Input: part model. Units: mm. Frame: model coordinates. A direction names the side the tool comes from. Coordinates: 2 decimals unless noted, no trailing zeros. Order: outer loops, then holes, each group sorted by start corner. A loop starts at its lowest first (then second) coordinate and runs counter-clockwise, first axis right, second up. Notation, with made-up numbers: (-13.5, -27) -> (21.5, -27) arc R13 ccw to (21.5, -21) -> close; hole circle Ø5 at (47, 39). An arc over 180 degrees is marked (long way). Use one line per item in the form item = value. Start each with the question number.
1) Ray query, line 1 along X through (y, z) = (54, 203); line 2 along Z through (x, y) = (-20, 92); line 3 along Y through (x, z) = (-42.5, -67). Return the intervals inside material, ascending.
2) Pin query (flat end, axial travel): pin 1 (15 mm diameter, centred on x = 118.06, z = -176.69, fed in from +Y); pin 2 (15 mm diameter, centred on x = -41.46, z = 208.42, fed in from -Y); pin 3 (1 mm diameter, centred on y = -22, z = -51, fed in from -X); pin 4 (10.5 mm diameter, centred on x = -41.46, z = -208.42, fed in from +Y). Return the tip coordinate at first contact, or that it passes through.
3) Access query for faces 4 (the flat face through (-188.79, 53.307, -105.435)), 5 (the conical face through (-81.465, 47.154, -197.721)), 6 (the cylindrical face through (-143.719, 61.042, 143.366)), 7 (the flat face through (105.7, 53.31, 188.99)). Directions: +Z, -Z, +X, -X, +Y, -Y. A direction counts if a zero-diameter tool reaches every point of the face in a straight line with its end or side. Return the directions, or none.
4) Section query C-C on y = 101. Output: boundary loops of the cut face in (x, z), then the cut area to 3 significant figures.
5) Draft query along X for faces 1 (the cylindrical face through (-187.452, 61.042, -77.915)), 2 (the conical face through (197.721, 47.154, -81.465)), 3 (the conical face through (0, 47, 214)). Return one class per face: pulls with the +X half, pulls with the -X half, needs draft (parallel to the pull), parting line crosses it, or undercut.
from build123d import *

# Parameters (mm, degrees)
CUT_EXTRUDE1_DEPTH = 28
CIRPATTERN1_COUNT  = 16
SKETCH5_R          = 6.5
CUT_EXTRUDE2_DEPTH = 336.079515181
CHAMFER1_SIZE      = 2


with BuildPart() as part:
    # Sketch1 → Revolve1 (revolve)
    with BuildSketch(Plane.XY, mode=Mode.PRIVATE) as revolve1_sk:
        Polygon((225, 0), (225, 64), (202.5, 64), (200, 95.5), (180, 95.5), (180, 123.5), (143, 123.5), (143, 88.5), (85, 88.5), (85, 116.5), (66, 116.5), (66, -41.015625), (86.5078125, -41.015625), (86.5078125, 0), align=None)
    revolve(revolve1_sk.sketch.rotate(Axis((0, 0, 0), (0, 1, 0)), 90), axis=Axis((0, 0, 0), (0, 1, 0)))

    # Sketch3 → Cut-Extrude1 (cut)
    with BuildSketch(Plane(origin=(0, 64, 0), x_dir=(1, 0, 0), z_dir=(0, 1, 0))):
        with BuildLine():
            Line((222.99103121, 30), (201.742410018, 17.5))
            ThreePointArc((201.742410018, 17.5), (202.5, 0), (201.742410018, -17.5))
            Line((201.742410018, -17.5), (222.99103121, -30))
            ThreePointArc((222.99103121, -30), (225, 0), (222.99103121, 30))
        make_face()
    cut_extrude1 = extrude(amount=-CUT_EXTRUDE1_DEPTH, mode=Mode.SUBTRACT)

    # CirPattern1: Cut-Extrude1 ×16 about axis
    cirpattern1_axis = Axis((0, 0, 0), (0, 1, 0))
    for i in range(1, CIRPATTERN1_COUNT):
        add(cut_extrude1.rotate(cirpattern1_axis, i * 360 / CIRPATTERN1_COUNT), mode=Mode.SUBTRACT)

    # Sketch4 → Revolve2 (revolve)
    with BuildSketch(Plane.XY):
        Polygon((225, 36), (203, 58), (203, 64), (195, 64), (195, 0), (225, 0), align=None)
    revolve(axis=Axis((0, 0, 0), (0, 1, 0)))

    # Sketch5 → Cut-Extrude2 (cut, through all)
    with BuildSketch(Plane(origin=(0, 64, 0), x_dir=(1, 0, 0), z_dir=(0, 1, 0))):
        with Locations(Location((208.416872086, 41.456693428, 0), (0, 0, 270))):
            Circle(SKETCH5_R)
        with Locations(Location((208.416872086, -41.456693428, 0), (0, 0, 270))):
            Circle(SKETCH5_R)
        with Locations(Location((176.687292614, -118.058674517, 0), (0, 0, 270))):
            Circle(SKETCH5_R)
        with Locations(Location((118.058674517, -176.687292614, 0), (0, 0, 270))):
            Circle(SKETCH5_R)
        with Locations(Location((41.456693428, -208.416872086, 0), (0, 0, 270))):
            Circle(SKETCH5_R)
        with Locations(Location((-41.456693428, -208.416872086, 0), (0, 0, 270))):
            Circle(SKETCH5_R)
        with Locations(Location((-118.058674517, -176.687292614, 0), (0, 0, 270))):
            Circle(SKETCH5_R)
        with Locations(Location((-176.687292614, -118.058674517, 0), (0, 0, 270))):
            Circle(SKETCH5_R)
        with Locations(Location((-208.416872086, -41.456693428, 0), (0, 0, 270))):
            Circle(SKETCH5_R)
        with Locations(Location((-208.416872086, 41.456693428, 0), (0, 0, 270))):
            Circle(SKETCH5_R)
        with Locations(Location((-176.687292614, 118.058674517, 0), (0, 0, 270))):
            Circle(SKETCH5_R)
        with Locations(Location((-118.058674517, 176.687292614, 0), (0, 0, 270))):
            Circle(SKETCH5_R)
        with Locations(Location((-41.456693428, 208.416872086, 0), (0, 0, 270))):
            Circle(SKETCH5_R)
        with Locations(Location((41.456693428, 208.416872086, 0), (0, 0, 270))):
            Circle(SKETCH5_R)
        with Locations(Location((118.058674517, 176.687292614, 0), (0, 0, 270))):
            Circle(SKETCH5_R)
        with Locations(Location((176.687292614, 118.058674517, 0), (0, 0, 270))):
            Circle(SKETCH5_R)
    extrude(amount=-CUT_EXTRUDE2_DEPTH, mode=Mode.SUBTRACT)

    # Chamfer1
    chamfer1_edges = [part.edges().sort_by_distance(p)[0] for p in [
        (0, 0, 225),
    ]]
    chamfer(chamfer1_edges, length=CHAMFER1_SIZE)


solid = part.part
Answers below:
q1.line_1 = -59.65 to -45.05, -37.86 to 37.86, 45.05 to 59.65
q1.line_2 = -199.28 to -141.59, -82.61 to -62.9, 62.9 to 82.61, 141.59 to 199.28
q1.line_3 = -41.02 to 116.5
q2.pin_1 = 64
q2.pin_2 = 0
q2.pin_3 = -70.24
q2.pin_4 = through
q3.face_4 = -X, +Y
q3.face_5 = -Z, +Y
q3.face_6 = +Y
q3.face_7 = +Z, +Y
q4.outline = circle Ø360 at (0, 0); circle Ø170 at (0, 0); hole circle Ø286 at (0, 0); hole circle Ø132 at (0, 0)
q4.area = 46,600 mm^2
q5.face_1 = pulls with the -X half
q5.face_2 = pulls with the +X half
q5.face_3 = undercut
